```python
from build123d import *

# Parameters (mm, degrees)
F0_W     = 52.234799
F0_H     = 96.570488
F1_DEPTH = 25.4
F2_R     = 5.08
F3_W     = 21.627817
F3_H     = 31.183585
F4_DEPTH = 8.342061


with BuildPart() as f1:
    # F0 (on Top) → F1 (new body)
    with BuildSketch(Plane.XY):
        with Locations((26.117399, -1.483681)):
            Rectangle(F0_W, F0_H)
    extrude(amount=F1_DEPTH)

    # F2
    f2_edges = [f1.edges().sort_by_distance(p)[0] for p in [
        (52.234799, -1.483681, 25.4),
    ]]
    fillet(f2_edges, radius=F2_R)

    # F3 (on face) → F4 (join)
    with BuildSketch(Plane.XY.offset(25.4)):
        with Locations((28.650353, -9.590007)):
            Rectangle(F3_W, F3_H)
    extrude(amount=F4_DEPTH)


solid = f1.part
```
The listing builds one solid part. Answer for the finished solid, in the listing's coordinates (mm). A direction names the side the tool comes from. Give positions to 0.01 mm unless a question says otherwise; leave off trailing zeros. Order: outer loops, then holes, each group sorted by start corner. A loop starts at its lowest first (then second) coordinate and runs counter-clockwise, first axis right, second up. Notation, with made-up numbers: (31.25, 27.25) -> (39.25, 27.25) arc R21 cw to (39.25, 31.25) -> close; hole circle Ø10 at (21.5, 61.5). An arc over 180 degrees is marked (long way). Answer as CSV lines item,"result". Start each with the question number.
Q1. A cutting plane is placed at B-B (y = -10). Determine the outline of the cut face in (x, z), then the cut area to 3 significant figures.
Q2. A cutting plane is placed at C-C (z = 30.5). Determine the outline of the cut face in (x, y), then the cut area to 3 significant figures.
Q3. A cutting plane is placed at A-A (x = 19). Determine the outline of the cut face in (y, z).
Q4. Given pin 1 (4 mm diameter, centred on x = 24.5, z = 29.5, fed in from +Y); pin 2 (9 mm diameter, centred on y = -5, z = 29, fed in from +X); pin 3 (4 mm diameter, centred on x = 24.5, z = 31, fed in from -Y), each flat-ended and moving along its own axis, determine where each tip first touches the part or whether it passes through.
Q5. Which of the six approach directions +Z, -Z, +X, -X, +Y, -Y give full straight-line access (tool end or side, diameter ignored) to faces 1 (the flat face through (39.464, -10, 30)), 2 (the flat face through (17.836, -10, 30)), 3 (the flat face through (28, 6.002, 30)), 4 (the flat face through (26, 46.802, 13)), 5 (the flat face through (28, -25.182, 30))?
Q6. A cutting plane is placed at D-D (y = 40). Determine the outline of the cut face in (x, z), then the cut area to 3 significant figures.
Q7. Find the intervals of material crossed by L1, parallel to Z at x = 3, y = -21; L2, parallel to X at y = -19.5, z = 31.5; L3, parallel to X at y = 43.5, z = 21.5, in increasing order.
Results found:
1,outline,"(0, 0) -> (52.23, 0) -> (52.23, 20.32) arc R5.08 ccw to (47.15, 25.4) -> (39.46, 25.4) -> (39.46, 33.74) -> (17.84, 33.74) -> (17.84, 25.4) -> (0, 25.4) -> close"
1,area,"1,500 mm2"
2,outline,"(17.84, -25.18) -> (39.46, -25.18) -> (39.46, 6) -> (17.84, 6) -> close"
2,area,"674 mm2"
3,outline,"(-49.77, 0) -> (46.8, 0) -> (46.8, 25.4) -> (6, 25.4) -> (6, 33.74) -> (-25.18, 33.74) -> (-25.18, 25.4) -> (-49.77, 25.4) -> close"
4,pin 1,"y = 6"
4,pin 2,"x = 50.04"
4,pin 3,"y = -25.18"
5,face 1,"+Z, +X, +Y, -Y"
5,face 2,"+Z, -X, +Y, -Y"
5,face 3,"+Z, +X, -X, +Y"
5,face 4,"+Z, -Z, +X, -X, +Y"
5,face 5,"+Z, +X, -X, -Y"
6,outline,"(0, 0) -> (52.23, 0) -> (52.23, 20.32) arc R5.08 ccw to (47.15, 25.4) -> (0, 25.4) -> close"
6,area,"1,320 mm2"
7,L1,"0 to 25.4"
7,L2,"17.84 to 39.46"
7,L3,"0 to 52.1"
